Geometry check sheet. Reference: the model listing, model coordinates, mm. Face numbers are marked on the shaded views. A direction names the side the tool comes from. Give positions to 0.01 mm unless a question says otherwise; leave off trailing zeros. Write each loop counter-clockwise with the first axis right and the second up, starting at its lowest first coordinate (ties: lowest second). Pieces come first, ordered by that corner, then holes. Notation, with made-up numbers: (82.5, 39) -> (113.5, 39) arc R18 ccw to (113.5, 74) -> close; hole circle Ø9 at (25.5, -2.5). An arc over 180 degrees is marked (long way). One line per item, written item: value.
from build123d import *

# Parameters (mm, degrees)
ESQUISSE1_R        = 2.5
BOSS_EXTRU_1_DEPTH = 10
ESQUISSE2_R        = 10
BOSS_EXTRU_2_DEPTH = 66
CONG_1_R           = 5.5


with BuildPart() as part:
    # Esquisse1 → Boss.-Extru.1 (new, symmetric)
    with BuildSketch(Plane.XY):
        with BuildLine():
            Line((5, 10), (5, -10))
            ThreePointArc((5, -10), (0, -15), (-5, -10))
            Line((-5, -10), (-5, 10))
            ThreePointArc((-5, 10), (0, 15), (5, 10))
        make_face()
        with Locations((0, 10)):
            Circle(ESQUISSE1_R, mode=Mode.SUBTRACT)
        with Locations((0, -10)):
            Circle(ESQUISSE1_R, mode=Mode.SUBTRACT)
    extrude(amount=BOSS_EXTRU_1_DEPTH, both=True)

    # Esquisse2 → Boss.-Extru.2 (add)
    with BuildSketch(Plane(origin=(5, 0, 0), x_dir=(0, 0, -1), z_dir=(1, 0, 0))):
        with Locations((0, 10)):
            Circle(ESQUISSE2_R)
    extrude(amount=BOSS_EXTRU_2_DEPTH)

    # Congé1
    cong_1_edges = [part.edges().sort_by_distance(p)[0] for p in [
        (71, 10, 10),
    ]]
    fillet(cong_1_edges, radius=CONG_1_R)


solid = part.part
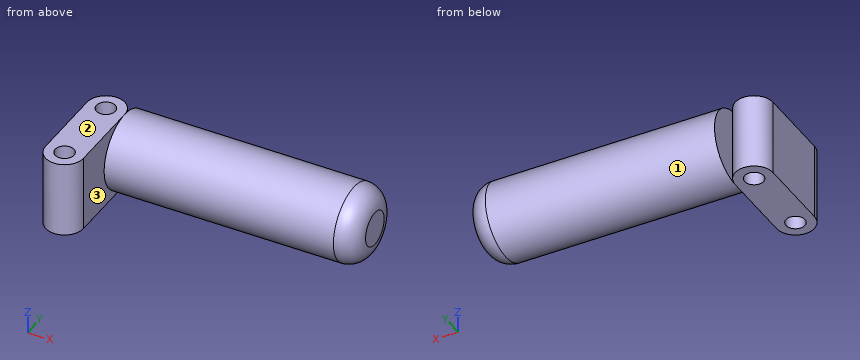
1) Tool access check on the marked faces 1, 2 and 3. Record the directions out of +Z, -Z, +X, -X, +Y, -Y that give a thin tool (end or side, any length) a straight path to the whole face; none if there is none.
Verdict:
face 1: +X
face 2: +Z, +X, -X, +Y, -Y
face 3: +X, -Y
2) Sectioned sample at D-D on y = -4. Record the cut outline in (x, z).
Verdict:
outline: (-5, -10) -> (5, -10) -> (5, 10) -> (-5, 10) -> close
3) Depth check by flat-ended pin: pin 1 Ø1 at (x, z) = (63, 5.5) entering from -Y; pin 2 Ø5 at (x, z) = (18.5, -0.5) entering from -Y; pin 3 Ø12 at (x, y) = (17, 1) entering from +Z. Enter the tip coordinate at first touch or a pass-through.
Verdict:
pin 1: y = 1.34
pin 2: y = 0
pin 3: z = 9.54
4) Sectioned sample at B-B on z = 0. Give the number of separate pieces and of enclosed holes in the cut face, plus the area to 3 significant figures.
Verdict:
separate pieces: 1
enclosed holes: 2
area: 1,550 mm^2
5) Sectioned sample at A-A on x = 0. Record the cut outline in (y, z), plus the area to 3 significant figures.
Verdict:
outline: (-15, -10) -> (-12.5, -10) -> (-12.5, 10) -> (-15, 10) -> close; (-7.5, -10) -> (7.5, -10) -> (7.5, 10) -> (-7.5, 10) -> close; (12.5, -10) -> (15, -10) -> (15, 10) -> (12.5, 10) -> close
area: 400 mm^2
6) Scan lines: probe 1 along Y at (x, z) = (0, 1); probe 2 along X at (y, z) = (-8.5, 8.5); probe 3 along Z at (x, y) = (21, 18). Record each from-to range of solid material in increasing order.
Verdict:
probe 1: -15 to -12.5, -7.5 to 7.5, 12.5 to 15
probe 2: -5 to -2, 2 to 5
probe 3: -6 to 6
